```python
from build123d import *

# Parameters (mm, degrees)
ESQUISSE1_W             = 3
ESQUISSE1_H             = 30
BOSS_EXTRU_1_DEPTH      = 41.27
ESQUISSE1_3_W           = 36
ESQUISSE1_3_H           = 30
BOSS_EXTRU_2_DEPTH      = 3
ESQUISSE3_R             = 2.5
ESQUISSE3_R_2           = 1.6
ENL_V_MAT_EXTRU_2_DEPTH = 85
CONG_2_R                = 2
CONG_3_R                = 10
ESQUISSE7_R             = 2.5
ESQUISSE7_R_2           = 1.75
ENL_V_MAT_EXTRU_3_DEPTH = 10
ESQUISSE8_W             = 23
ESQUISSE8_H             = 3
BOSS_EXTRU_3_DEPTH      = 3


with BuildPart() as part:
    # Esquisse1 → Boss.-Extru.1 (new body)
    with BuildSketch(Plane.XY):
        with Locations((34.5, 15)):
            Rectangle(ESQUISSE1_W, ESQUISSE1_H)
    extrude(amount=BOSS_EXTRU_1_DEPTH)

    # Esquisse1<3> → Boss.-Extru.2 (add)
    with BuildSketch(Plane.XY):
        with Locations((18, 15)):
            Rectangle(ESQUISSE1_3_W, ESQUISSE1_3_H)
    extrude(amount=-BOSS_EXTRU_2_DEPTH)

    # Esquisse3 → Enlèv. mat.-Extru.2 (cut)
    with BuildSketch(Plane(origin=(36, 0, 0), x_dir=(0, 0, -1), z_dir=(1, 0, 0))):
        with Locations((-30.197874881, 15)):
            Circle(ESQUISSE3_R)
        with Locations((-30.197874881, 22)):
            Circle(ESQUISSE3_R_2)
        with Locations((-30.197874881, 8)):
            Circle(ESQUISSE3_R_2)
    extrude(amount=-ENL_V_MAT_EXTRU_2_DEPTH, mode=Mode.SUBTRACT)

    # Congé2
    cong_2_edges = [part.edges().sort_by_distance(p)[0] for p in [
        (33, 15, 0),
    ]]
    fillet(cong_2_edges, radius=CONG_2_R)

    # Congé3
    cong_3_edges = [part.edges().sort_by_distance(p)[0] for p in [
        (34.5, 0, 41.27),
        (0, 0, -1.5),
        (0, 30, -1.5),
        (34.5, 30, 41.27),
    ]]
    fillet(cong_3_edges, radius=CONG_3_R)

    # Esquisse7 → Enlèv. mat.-Extru.3 (cut)
    with BuildSketch(Plane(origin=(0, 0, -3), x_dir=(-1, 0, 0), z_dir=(0, 0, -1))):
        with Locations((-18, 15)):
            Circle(ESQUISSE7_R)
        with Locations((-18, 23.5)):
            Circle(ESQUISSE7_R_2)
        with Locations((-18, 6.5)):
            Circle(ESQUISSE7_R_2)
    extrude(amount=-ENL_V_MAT_EXTRU_3_DEPTH, mode=Mode.SUBTRACT)

    # Esquisse8 → Boss.-Extru.3 (add)
    with BuildSketch(Plane.XY):
        with Locations((21.5, 28.5)):
            Rectangle(ESQUISSE8_W, ESQUISSE8_H)
        with Locations((21.5, 1.5)):
            Rectangle(ESQUISSE8_W, ESQUISSE8_H)
    extrude(amount=BOSS_EXTRU_3_DEPTH)


solid = part.part
```
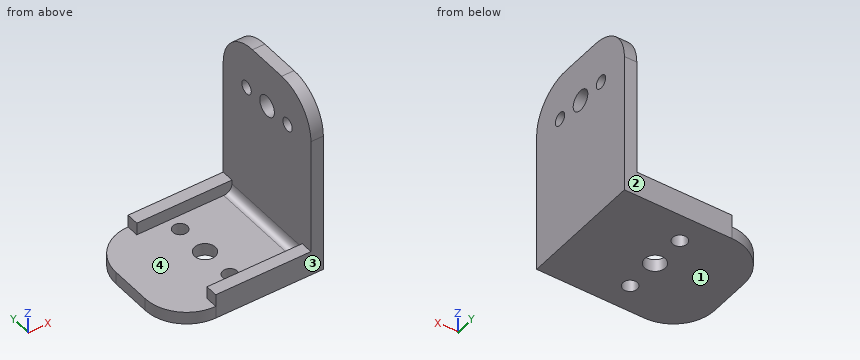
The listing builds one solid part. Answer for the finished solid, in the listing's coordinates (mm). Face numbers are marked on the shaded views. Give positions to 0.01 mm unless a question says otherwise; leave off trailing zeros. Write each loop counter-clockwise with the first axis right and the second up, starting at its lowest first coordinate (ties: lowest second). Pieces come first, ordered by that corner, then holes. Notation, with made-up numbers: (74.5, 88.5) -> (86.5, 88.5) arc R22 ccw to (86.5, 125.5) -> close; hole circle Ø6 at (30, -16). An arc over 180 degrees is marked (long way). Write item = value, one per line. Start each with the question number.
1) The part is cut by section A-A, the plane y = 15. Determine the outline of the cut face in (x, z).
2) The part is cut by section D-D, the plane y = 5.5. Determine the outline of the cut face in (x, z).
3) Determine the mould class of the marked faces 1, 2, 3 and 4 for opening direction Y: +Y half, -Y half, draft (parallel to the pull), parting line (faces both ways), or undercut.
4) The part is cut by section B-B, the plane x = 30. Determine the outline of the cut face in (y, z).
5) Each of these flat-tipped pins is pushed along its axis until it touches: pin 1 (1 mm diameter, centred on y = 6, z = 17, fed in from -X); pin 2 (4.5 mm diameter, centred on x = 18, y = 23.5, fed in from +Z); pin 3 (8 mm diameter, centred on x = 30, y = 3.5, fed in from +Z); pin 4 (4 mm diameter, centred on x = 30.5, z = 26.5, fed in from +Y). Where does it stop, or does it pass through?
6) Straight lines are drawn through the part: line 1 along Y through (x, z) = (18, -1); line 2 along X through (y, z) = (12, 8); line 3 along Z through (x, y) = (13, 7). For each, find the intervals that lie inside material, in ascending order.
7) The part is cut by section C-C, the plane z = 30.5. Determine the outline of the cut face in (x, y), and give its area (3 significant figures).
Solutions:
q1.outline = (0, -3) -> (15.5, -3) -> (15.5, 0) -> (0, 0) -> close; (20.5, -3) -> (36, -3) -> (36, 27.7) -> (33, 27.7) -> (33, 2) arc R2 cw to (31, 0) -> (20.5, 0) -> close; (33, 32.7) -> (36, 32.7) -> (36, 41.27) -> (33, 41.27) -> close
q2.outline = (1.07, -3) -> (16.56, -3) -> (16.56, 0) -> (1.07, 0) -> close; (19.44, -3) -> (36, -3) -> (36, 40.2) -> (33, 40.2) -> (33, 2) arc R2 cw to (31, 0) -> (19.44, 0) -> close
q3.face_1 = draft
q3.face_2 = +Y half
q3.face_3 = -Y half
q3.face_4 = undercut
q4.outline = (0, -3) -> (30, -3) -> (30, 3) -> (27, 3) -> (27, 0) -> (3, 0) -> (3, 3) -> (0, 3) -> close
q5.pin_1 = 33
q5.pin_2 = 0
q5.pin_3 = 40.5
q5.pin_4 = through
q6.line_1 = 0 to 4.75, 8.25 to 12.5, 17.5 to 21.75, 25.25 to 30
q6.line_2 = 33 to 36
q6.line_3 = -3 to 0
q7.outline = (33, 0) -> (36, 0) -> (36, 6.43) -> (33, 6.43) -> close; (33, 9.57) -> (36, 9.57) -> (36, 12.52) -> (33, 12.52) -> close; (33, 17.48) -> (36, 17.48) -> (36, 20.43) -> (33, 20.43) -> close; (33, 23.57) -> (36, 23.57) -> (36, 30) -> (33, 30) -> close
q7.area = 56.3 mm²
